from build123d import *

# Parameters (mm, degrees)
BOSS_EXTRUDE1_DEPTH                  = 79
SKETCH2_W                            = 72
SKETCH2_H                            = 2
BOSS_EXTRUDE2_DEPTH                  = 43
BOSS_EXTRUDE2_DIRECTION_2_REACH      = 99.642
BOSS_EXTRUDE2_DIRECTION_2_END_RADIUS = 36
SKETCH3_R                            = 1.3
CUT_EXTRUDE1_DEPTH                   = 10
SKETCH4_R                            = 1.3
CUT_EXTRUDE2_DEPTH                   = 118.753980824
FILLET1_R                            = 7


with BuildPart() as part:
    # Sketch1 → Boss-Extrude1 (new body)
    with BuildSketch(Plane.XY):
        with BuildLine():
            Line((-36, 0), (-36, -43))
            Line((-36, -43), (-38, -43))
            Line((-38, -43), (-38, 0))
            ThreePointArc((-38, 0), (0, 38), (38, 0))
            Line((38, 0), (38, -43))
            Line((38, -43), (36, -43))
            Line((36, -43), (36, 0))
            ThreePointArc((36, 0), (0, 36), (-36, 0))
        make_face()
    extrude(amount=BOSS_EXTRUDE1_DEPTH)

    # Sketch2 → Boss-Extrude2 (add)
    with BuildSketch(Plane(origin=(0, 0, 0), x_dir=(1, 0, 0), z_dir=(0, 1, 0))):
        with Locations((0, -78)):
            Rectangle(SKETCH2_W, SKETCH2_H)
    extrude(amount=-BOSS_EXTRUDE2_DEPTH)

    # Boss-Extrude2 direction 2: up to this cylinder (the profile starts inside it)
    boss_extrude2_direction_2_end = Plane(origin=(0, 0, 78), z_dir=(0, 0, -1)) * Cylinder(BOSS_EXTRUDE2_DIRECTION_2_END_RADIUS, 272.284, mode=Mode.PRIVATE)
    # Sketch2 → Boss-Extrude2 direction 2 (add, up to the surface)
    with BuildSketch(Plane(origin=(0, 0, 0), x_dir=(1, 0, 0), z_dir=(0, 1, 0)), mode=Mode.PRIVATE) as boss_extrude2_direction_2_sk1:
        with Locations((0, -78)):
            Rectangle(SKETCH2_W, SKETCH2_H)
    boss_extrude2_direction_2_tool1 = extrude(boss_extrude2_direction_2_sk1.sketch, amount=BOSS_EXTRUDE2_DIRECTION_2_REACH, mode=Mode.PRIVATE) & boss_extrude2_direction_2_end
    add(boss_extrude2_direction_2_tool1.solids().sort_by_distance((0, 0, 78))[0])

    # Sketch3 → Cut-Extrude1 (cut)
    with BuildSketch(Plane.XY.offset(79)):
        with Locations((-27.9, -39)):
            Circle(SKETCH3_R)
        with Locations((27.9, -39)):
            Circle(SKETCH3_R)
    extrude(amount=-CUT_EXTRUDE1_DEPTH, mode=Mode.SUBTRACT)

    # Sketch4 → Cut-Extrude2 (cut, through all)
    with BuildSketch(Plane(origin=(38, 0, 0), x_dir=(0, 0, -1), z_dir=(1, 0, 0))):
        with Locations(Location((-9.1, -39, 0), (0, 0, 90))):
            Circle(SKETCH4_R)
    extrude(amount=-CUT_EXTRUDE2_DEPTH, mode=Mode.SUBTRACT)

    # Fillet1
    fillet1_edges = [part.edges().sort_by_distance(p)[0] for p in [
        (-37, -43, 0),
        (37, -43, 0),
    ]]
    fillet(fillet1_edges, radius=FILLET1_R)


solid = part.part
Read the model definition and answer for the solid it produces. Units are mm, in the model's axes. A direction names the side the tool comes from. Round coordinates to 2 decimals unless told otherwise and drop trailing zeros. Write each loop counter-clockwise with the first axis right and the second up, starting at its lowest first coordinate (ties: lowest second). Pieces come first, ordered by that corner, then holes.
1. Which of the six approach directions +Z, -Z, +X, -X, +Y, -Y give full straight-line access (tool end or side, diameter ignored) to faces 1 (the face through (38, -21, 39)), 2 (the face through (-36, -21, 38))?
2. The part is cut by section A-A, the plane z = 9.1. Determine the outline of the cut face in (x, y), then the cut area to 3 significant figures.
3. Determine the mould class of faces 3 (the face through (-27.201, -37.904, 78.014)), 4 (the face through (37, -41, 2.1)), 5 (the face through (-0.84, 37.99, 38.95)) for opening direction X: pulls with the +X half, pulls with the -X half, needs draft (parallel to the pull), parting line crosses it, or undercut.
4. The part is cut by section C-C, the plane x = 27.9. Determine the outline of the cut face in (y, z), then the cut area to 3 significant figures.
5. The part is cut by section D-D, the plane y = -4.5. Determine the outline of the cut face in (x, z).
6. The part is cut by section B-B, the plane y = -39. Determine the outline of the cut face in (x, z).
7. Given pin 1 Ø10 at (y, z) = (0.5, 56) entering from +X; pin 2 Ø10 at (y, z) = (9, 33) entering from +X; pin 3 Ø12 at (x, z) = (12.5, 36) entering from +Y; pin 4 Ø1.5 at (x, z) = (17, 41) entering from -Y, each flat-ended and moving along its own axis, determine where each tip first touches the part or whether it passes through.
8. Straight lines are drawn through the part: L1, parallel to X at y = -15.5, z = 29.5; L2, parallel to Z at x = -19.5, y = -24.5; L3, parallel to Y at x = -27, z = 78. For each, find the intervals that lie inside material, in ascending order.
Values:
1. face 1: +Z, -Z, +X, +Y, -Y
1. face 2: -Z, -Y
2. outline: (-38, -43) - (-36, -43) - (-36, -40.3) - (-38, -40.3) - close; (-38, -37.7) - (-36, -37.7) - (-36, 0) arc R36 cw to (36, 0) - (36, -37.7) - (38, -37.7) - (38, 0) arc R38 ccw to (-38, 0) - close; (36, -43) - (38, -43) - (38, -40.3) - (36, -40.3) - close
2. area: 394 mm2
3. face 3: undercut
3. face 4: needs draft
3. face 5: parting line crosses it
4. outline: (-43, 77) - (-40.3, 77) - (-40.3, 79) - (-43, 79) - close; (-37.7, 77) - (22.75, 77) - (22.75, 0) - (25.8, 0) - (25.8, 79) - (-37.7, 79) - close
4. area: 367 mm2
5. outline: (-38, 0) - (-36, 0) - (-36, 77) - (36, 77) - (36, 0) - (38, 0) - (38, 79) - (-38, 79) - close
6. outline: (-38, 0.68) - (-36, 0.68) - (-36, 7.8) - (-38, 7.8) - close; (-38, 10.4) - (-36, 10.4) - (-36, 77) - (-29.2, 77) - (-29.2, 79) - (-38, 79) - close; (-26.6, 77) - (26.6, 77) - (26.6, 79) - (-26.6, 79) - close; (29.2, 77) - (36, 77) - (36, 10.4) - (38, 10.4) - (38, 79) - (29.2, 79) - close; (36, 0.68) - (38, 0.68) - (38, 7.8) - (36, 7.8) - close
7. pin 1: stops at x = 38
7. pin 2: stops at x = 37.79
7. pin 3: stops at y = 37.44
7. pin 4: stops at y = 31.32
8. L1: x = -38 to -36, 36 to 38
8. L2: z = 77 to 79
8. L3: y = -43 to -39.94, -38.06 to 26.74
